Verification items for the finished model (mm, model axes). A direction names the side the tool comes from. Coordinates: 2 decimals unless noted, no trailing zeros. Write each loop counter-clockwise with the first axis right and the second up, starting at its lowest first coordinate (ties: lowest second). Pieces come first, ordered by that corner, then holes. Notation, with made-up numbers: (75.5, -3) - (83.5, -3) arc R30 ccw to (83.5, 22) - close; hole circle Ø7 at (79, 22). An arc over 180 degrees is marked (long way). Answer as CSV lines item,"result". Start each with the question number.
```python
from build123d import *

# Parameters (mm, degrees)
BOSS_EXTRUDE1_DEPTH   = 4.6
M5X0_8_TAPPED_HOLE1_D = 4.2
FILLET1_R             = 4.25
SKETCH9_R             = 8.7
BOSS_EXTRUDE2_DEPTH   = 43.7
SKETCH10_R            = 4.7625
CUT_EXTRUDE1_DEPTH    = 48.3


with BuildPart() as part:
    # Sketch1 → Boss-Extrude1 (new body)
    with BuildSketch(Plane.XY):
        Polygon((0, 23.094010768), (20, -11.547005384), (-20, -11.547005384), align=None)
    extrude(amount=BOSS_EXTRUDE1_DEPTH)

    # M5x0.8 Tapped Hole1 (through all)
    with Locations(Plane(origin=(0, 0, 0), x_dir=(-1, 0, 0), z_dir=(0, 0, -1))):
        with Locations((0, 14.594010768), (-12.5, -7.056624327), (12.5, -7.056624327)):
            Hole(M5X0_8_TAPPED_HOLE1_D / 2)

    # Fillet1
    fillet1_edges = [part.edges().sort_by_distance(p)[0] for p in [
        (0, 23.094010768, 2.3),
        (20, -11.547005384, 2.3),
        (-20, -11.547005384, 2.3),
    ]]
    fillet(fillet1_edges, radius=FILLET1_R)

    # Sketch9 → Boss-Extrude2 (add)
    with BuildSketch(Plane(origin=(0, 0, 0), x_dir=(-1, 0, 0), z_dir=(0, 0, -1))):
        Circle(SKETCH9_R)
    extrude(amount=BOSS_EXTRUDE2_DEPTH)

    # Sketch10 → Cut-Extrude1 (cut)
    with BuildSketch(Plane(origin=(0, 0, -43.7), x_dir=(-1, 0, 0), z_dir=(0, 0, -1))):
        Circle(SKETCH10_R)
    extrude(amount=-CUT_EXTRUDE1_DEPTH, mode=Mode.SUBTRACT)


solid = part.part
```
1. Cross-section at A-A (x = 0). Record the cut outline in (y, z), and give its area (3 significant figures).
2. Cross-section at C-C (z = -29). Record the cut outline in (x, y) (1 decimal), and give its area (3 significant figures).
3. Cross-section at D-D (x = 12). Record the cut outline in (y, z).
4. Access from +Z, -Z, +X, -X, +Y, -Y to the whole of each face (thin tool, end or side, straight path). Record for faces 5 (the face through (0.062, 18.844, 2.332)), 6 (the face through (1, -9, 0)).
5. Cross-section at B-B (y = 1). Record the cut outline in (x, z), and give its area (3 significant figures).
6. Draft check along Y on faces 1 (the face through (3.78, -2.9, -19.89)), 2 (the face through (16.35, -9.37, 2.33)), 3 (the face through (0, -11.547, 2)), 4 (the face through (10.95, -5.64, 2.33)). Enter one of: pulls with the +Y half, pulls with the -Y half, needs draft (parallel to the pull), parting line crosses it, or undercut.
7. Depth check by flat-ended pin: P1, Ø1.5, axis at x = -7, z = -16, coming from the +Y side; P2, Ø3, axis at y = -4.5, z = -7.5, coming from the -X side; P3, Ø1, axis at y = 6.5, z = -19, coming from the -X side. Enter the tip coordinate at first touch or a pass-through.
8. Scan lines: line 1 along Y through (x, z) = (0, -23); line 2 along X through (y, z) = (-1, -2); line 3 along X through (y, z) = (3, -22.5). Record each from-to range of solid material in increasing order. Write a range as from..to.
Completed:
1,outline,"(-11.55, 0) - (-8.7, 0) - (-8.7, -43.7) - (-4.76, -43.7) - (-4.76, 4.6) - (-11.55, 4.6) - close; (4.76, -43.7) - (8.7, -43.7) - (8.7, 0) - (12.49, 0) - (12.49, 4.6) - (4.76, 4.6) - close; (16.69, 0) - (18.84, 0) - (18.84, 4.6) - (16.69, 4.6) - close"
1,area,"421 mm2"
2,outline,"circle Ø17.4 at (0, 0); hole circle Ø9.5 at (0, 0)"
2,area,"167 mm2"
3,outline,"(-11.55, 0) - (-9.1, 0) - (-9.1, 4.6) - (-11.55, 4.6) - close; (-5.02, 0) - (2.31, 0) - (2.31, 4.6) - (-5.02, 4.6) - close"
4,face 5,"+Z, -Z, +Y"
4,face 6,"-Z"
5,outline,"(-12.76, 0) - (-8.64, 0) - (-8.64, -43.7) - (-4.66, -43.7) - (-4.66, 4.6) - (-12.76, 4.6) - close; (4.66, -43.7) - (8.64, -43.7) - (8.64, 0) - (12.76, 0) - (12.76, 4.6) - (4.66, 4.6) - close"
5,area,"423 mm2"
6,face 1,"undercut"
6,face 2,"parting line crosses it"
6,face 3,"pulls with the -Y half"
6,face 4,"undercut"
7,P1,"stops at y = 6.05"
7,P2,"stops at x = -8.17"
7,P3,"stops at x = -6.3"
8,line 1,"y = -8.7..-4.76, 4.76..8.7"
8,line 2,"x = -8.64..-4.66, 4.66..8.64"
8,line 3,"x = -8.17..-3.7, 3.7..8.17"
